Verification items for this drawing (mm, ordinates from the low corner). Round coordinates to 2 decimals unless told otherwise and drop trailing zeros. Order: outer loops, then holes, each group sorted by start corner. A loop starts at its lowest first (then second) coordinate and runs counter-clockwise, first axis right, second up.
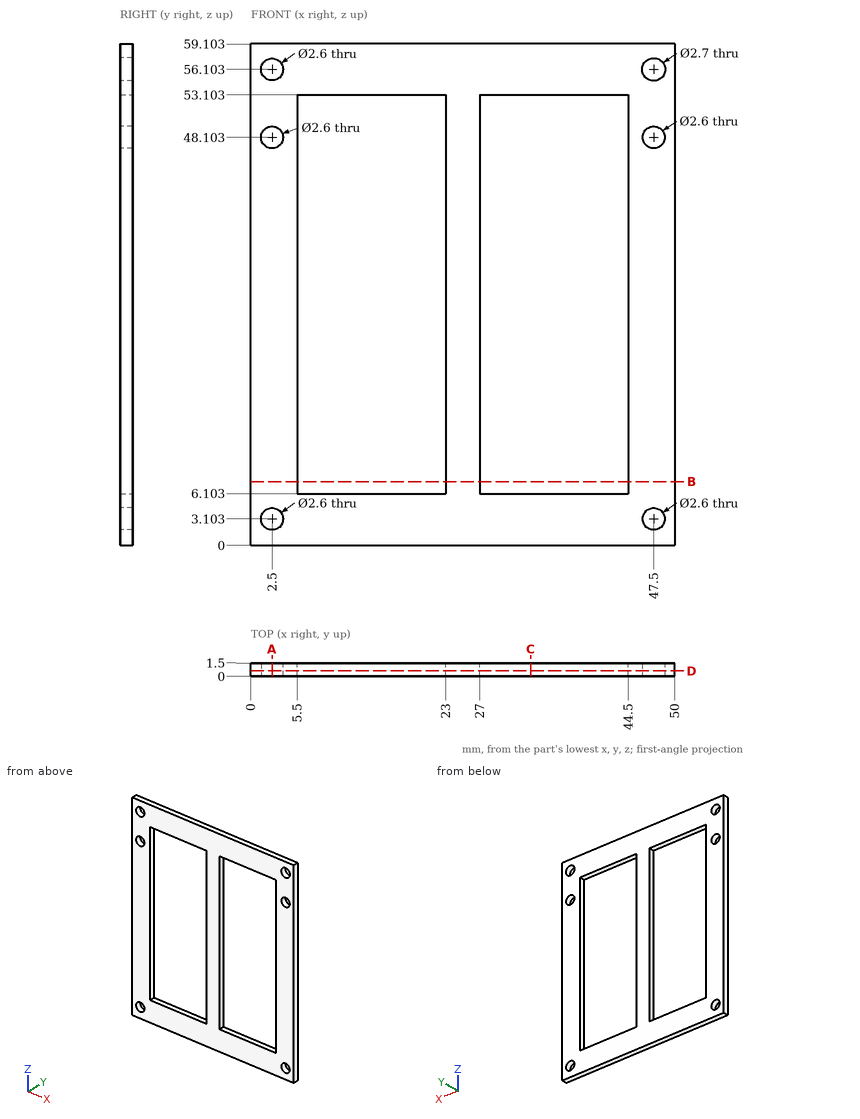
Item 1: Go/stop test with a flat-tipped pin: P1, Ø1.6, axis at x = 47.5, z = 48.1, coming from the +Y side. Record where the tip stops, or that it passes through.
Answer:
P1: passes through
Item 2: Sectioned sample at A-A (x = 2.5). Record the cut outline in (y, z).
Answer:
outline: (0, 0) - (1.5, 0) - (1.5, 1.8) - (0, 1.8) - close; (0, 4.4) - (1.5, 4.4) - (1.5, 46.8) - (0, 46.8) - close; (0, 49.4) - (1.5, 49.4) - (1.5, 54.8) - (0, 54.8) - close; (0, 57.4) - (1.5, 57.4) - (1.5, 59.1) - (0, 59.1) - close
Item 3: Sectioned sample at D-D (y = 0.6). State how many separate pieces and enclosed holes the cut face has, and give its area (3 significant figures).
Answer:
separate pieces: 1
enclosed holes: 8
area: 1,280 mm2
Item 4: Sectioned sample at B-B (z = 7.5). Record the cut outline in (x, y).
Answer:
outline: (0, 0) - (5.5, 0) - (5.5, 1.5) - (0, 1.5) - close; (23, 0) - (27, 0) - (27, 1.5) - (23, 1.5) - close; (44.5, 0) - (50, 0) - (50, 1.5) - (44.5, 1.5) - close
Item 5: Sectioned sample at C-C (x = 33). Record the cut outline in (y, z).
Answer:
outline: (0, 0) - (1.5, 0) - (1.5, 6.1) - (0, 6.1) - close; (0, 53.1) - (1.5, 53.1) - (1.5, 59.1) - (0, 59.1) - close
Item 6: Scan lines: line 1 along X through (y, z) = (1.05, 42); line 2 along Z through (x, y) = (2.5, 0.7); line 3 along Z through (x, y) = (47.5, 0.8). Record each from-to range of solid material in increasing order.
Answer:
line 1: x = 0 to 5.5, 23 to 27, 44.5 to 50
line 2: z = 0 to 1.8, 4.4 to 46.8, 49.4 to 54.8, 57.4 to 59.1
line 3: z = 0 to 1.8, 4.4 to 46.8, 49.4 to 54.75, 57.45 to 59.1
